Source: CAD feature listing. Evaluate the final solid. Frame: model axes, mm. A direction names the side the tool comes from. Give positions to 0.01 mm unless a question says otherwise; leave off trailing zeros. Order: outer loops, then holes, each group sorted by start corner. A loop starts at its lowest first (then second) coordinate and runs counter-clockwise, first axis right, second up. Notation, with made-up numbers: (82.25, -11) - (127.25, -11) arc R15 cw to (127.25, 7) - close; hole circle Ø10 at (49.5, 53.25). An arc over 180 degrees is marked (long way). One line per item, written item: value. Start each with the question number.
from build123d import *

# Parameters (mm, degrees)
SKETCH1_W = 100
SKETCH1_H = 100


with BuildPart() as part:
    # Sweep1: sweep along a path in Sketch3
    with BuildLine(Plane(origin=(0, 0, 0), x_dir=(0, 0, -1), z_dir=(1, 0, 0))) as sweep1_path:
        Line((0, 0), (120, 0))
        Line((120, 0), (176.568542495, 56.568542495))
        Line((176.568542495, 56.568542495), (206.151820817, 120.010087587))
    # Sketch1 → Sweep1 (sweep)
    with BuildSketch(Plane.XY):
        Rectangle(SKETCH1_W, SKETCH1_H)
    sweep(path=sweep1_path.line, transition=Transition.RIGHT)


solid = part.part
1. Set-up query: faces 1 (the flat face through (-1, -50, -71)), 2 (the flat face through (1, 50, -50)). Return all of +Z, -Z, +X, -X, +Y, -Y with unobstructed straight access to the full face (end or side cutting, diameter ignored); none if empty.
2. Section B-B on z = -81.5. Return the cut outline in (x, y), then the cut area to 3 significant figures.
3. Section C-C on y = 42.5. Return the cut outline in (x, z).
4. Contact query for flat-ended pins moving along their axis: pin 1 Ø10 at (x, y) = (-1.5, 6.5) entering from +Z; pin 2 Ø5 at (x, y) = (37.5, 92) entering from +Z; pin 3 Ø1 at (x, z) = (12, -160) entering from -Y. Output: stop coordinate, or through.
5. Ray query, L1, parallel to Y at x = -43.5, z = -95; L2, parallel to Z at x = 5.5, y = 35; L3, parallel to Z at x = 39, y = 110. Return the intervals inside material, ascending.
6. Section A-A on x = 12.5. Return the cut outline in (y, z), then the cut area to 3 significant figures.
Data:
1. face 1: +Z, -Z, +X, -X, -Y
1. face 2: +Z, +X, -X, +Y
2. outline: (-50, -50) - (50, -50) - (50, 50) - (-50, 50) - close
2. area: 10,000 mm2
3. outline: (-50, -225.18) - (50, -225.18) - (50, 0) - (-50, 0) - close
4. pin 1: stops at z = 0
4. pin 2: stops at z = -136.76
4. pin 3: stops at y = -31.21
5. L1: y = -50 to 50
5. L2: z = -221.68 to 0
5. L3: z = -227.62 to -146.32
6. outline: (-50, -140.71) - (27.45, -218.16) - (98.88, -251.47) - (141.14, -160.84) - (85.69, -134.98) - (50, -99.29) - (50, 0) - (-50, 0) - close
6. area: 27,000 mm2
